Input: part model. Units: mm. Frame: model coordinates. Face numbers are marked on the shaded views. A direction names the side the tool comes from. Round coordinates to 2 decimals unless told otherwise and drop trailing zeros. Loops run counter-clockwise (first coordinate to the right, second up) from the corner with the lowest first, then second, coordinate; pieces in that order, holes last. Notation, with made-up numbers: M -12,73 L 0,73 A36 cw 0,107 Z; hole C 28,66 d9. An arc over 180 degrees is marked long. Put each result on its own line as item: value. Start each with the question number.
1) Section C-C on x = 176.75. State how many separate pieces and enclosed holes the cut face has, plus the area to 3 significant figures.
2) Reachability of the marked faces 1 and 2 from +Z, -Z, +X, -X, +Y, -Y: full face, straight path, thin tool, end or side. Return the list, or none.
3) Section A-A on z = 1.5. Output: boundary loops of the cut face in (x, y), plus the area to 3 significant figures.
4) Line query: probe 1 along Y at (x, z) = (172, 5); probe 2 along Y at (x, z) = (174, 3.75); probe 3 along Z at (x, y) = (179.25, 60.5). Output: solid intervals per line, ascending.
5) Pin query (flat end, axial travel): pin 1 (6 mm diameter, centred on x = 173.5, z = 15, fed in from -Y); pin 2 (1.1 mm diameter, centred on x = 178, y = 59.5, fed in from +Z); pin 3 (1.1 mm diameter, centred on x = 176.5, y = 73.5, fed in from +Z); pin 4 (3 mm diameter, centred on y = 75.4, z = 14.15, fed in from -X). Return the tip coordinate at first contact, or that it passes through.
6) Section B-B on y = 59.5. Output: boundary loops of the cut face in (x, z).
7) Section D-D on z = 4. Output: boundary loops of the cut face in (x, y).
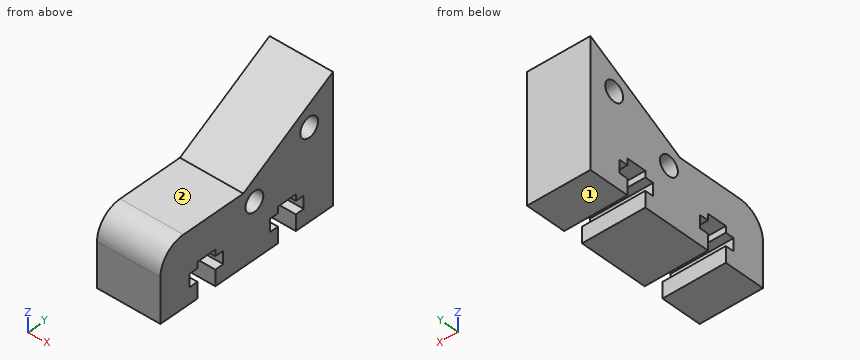
from build123d import *

# Parameters (mm, degrees)
SZKIC1_W                    = 10
SZKIC1_H                    = 30
DODANIE_WYCI_GNI_CIE1_DEPTH = 30
WYTNIJ_WYCI_GNI_CIE1_DEPTH  = 10
SZYK_LINIOWY1_COUNT         = 2
SZYK_LINIOWY1_PITCH         = 14
WYTNIJ_WYCI_GNI_CIE2_DEPTH  = 10
SZKIC7_R                    = 1.55
WYTNIJ_WYCI_GNI_CIE4_DEPTH  = 20
WYTNIJ_WYCI_GNI_CIE5_DEPTH  = 10


with BuildPart() as part:
    # Szkic1 → Dodanie-wyciągnięcie1 (new body)
    with BuildSketch(Plane.XY):
        with Locations((175.434880274, 64.530770571)):
            Rectangle(SZKIC1_W, SZKIC1_H)
    extrude(amount=DODANIE_WYCI_GNI_CIE1_DEPTH)

    # Szkic3 → Wytnij-wyciągnięcie1 (cut)
    with BuildSketch(Plane(origin=(180.434880274, 0, 0), x_dir=(0, 0, -1), z_dir=(1, 0, 0))):
        Polygon((0, 73.080770571), (0, 69.980770571), (-2.5, 69.980770571), (-2.5, 68.605770571), (-4.5, 68.605770571), (-4.5, 69.980770571), (-5.5, 69.980770571), (-5.5, 73.080770571), (-4.5, 73.080770571), (-4.5, 74.455770571), (-2.5, 74.455770571), (-2.5, 73.080770571), align=None)
    wytnij_wyci_gni_cie1 = extrude(amount=-WYTNIJ_WYCI_GNI_CIE1_DEPTH, mode=Mode.SUBTRACT)

    # Szyk liniowy1: Wytnij-wyciągnięcie1 ×2
    with Locations(*[(0, -i * SZYK_LINIOWY1_PITCH, 0) for i in range(1, SZYK_LINIOWY1_COUNT)]):
        add(wytnij_wyci_gni_cie1, mode=Mode.SUBTRACT)

    # Szkic4 → Wytnij-wyciągnięcie2 (cut)
    with BuildSketch(Plane(origin=(180.434880274, 0, 0), x_dir=(0, 0, -1), z_dir=(1, 0, 0))):
        Polygon((-20, 79.530770571), (-11, 63.942313303), (-11, 49.530770571), (-30, 49.530770571), (-30, 79.530770571), align=None)
    extrude(amount=-WYTNIJ_WYCI_GNI_CIE2_DEPTH, mode=Mode.SUBTRACT)

    # Szkic7 → Wytnij-wyciągnięcie4 (cut)
    with BuildSketch(Plane(origin=(180.434880274, 0, 0), x_dir=(0, 0, -1), z_dir=(1, 0, 0))):
        with Locations((-8.651923789, 65.875326005)):
            Circle(SZKIC7_R)
        with Locations((-14.151923789, 75.401605446)):
            Circle(SZKIC7_R)
    extrude(amount=-WYTNIJ_WYCI_GNI_CIE4_DEPTH, mode=Mode.SUBTRACT)

    # Szkic8 → Wytnij-wyciągnięcie5 (cut)
    with BuildSketch(Plane(origin=(180.434880274, 0, 0), x_dir=(0, 0, -1), z_dir=(1, 0, 0))):
        with BuildLine():
            Line((-7, 49.530770571), (-11, 49.530770571))
            Line((-11, 49.530770571), (-11, 53.530770571))
            ThreePointArc((-11, 53.530770571), (-9.828427125, 50.702343446), (-7, 49.530770571))
        make_face()
    extrude(amount=-WYTNIJ_WYCI_GNI_CIE5_DEPTH, mode=Mode.SUBTRACT)


solid = part.part
Geometry results:
1. separate pieces: 1
1. enclosed holes: 2
1. area: 337 mm²
2. face 1: -Z, +X, -X, +Y, -Y
2. face 2: +Z, +X, -X, -Y
3. outline: M 170.43,49.53 L 180.43,49.53 L 180.43,55.98 L 170.43,55.98 Z; M 170.43,59.08 L 180.43,59.08 L 180.43,69.98 L 170.43,69.98 Z; M 170.43,73.08 L 180.43,73.08 L 180.43,79.53 L 170.43,79.53 Z
3. area: 238 mm²
4. probe 1: y = 49.53 to 55.98, 59.08 to 69.98, 73.08 to 79.53
4. probe 2: y = 49.53 to 54.61, 60.46 to 68.61, 74.46 to 79.53
4. probe 3: z = 0 to 11
5. pin 1: stops at y = 65.67
5. pin 2: stops at z = 11
5. pin 3: stops at z = 16.84
5. pin 4: passes through
6. outline: M 170.43,0 L 180.43,0 L 180.43,2.5 L 170.43,2.5 Z; M 170.43,4.5 L 180.43,4.5 L 180.43,11 L 170.43,11 Z
7. outline: M 170.43,49.53 L 180.43,49.53 L 180.43,54.61 L 170.43,54.61 Z; M 170.43,60.46 L 180.43,60.46 L 180.43,68.61 L 170.43,68.61 Z; M 170.43,74.46 L 180.43,74.46 L 180.43,79.53 L 170.43,79.53 Z
